Drawing for the job (mm, zero at the part's lowest x, y, z). Round coordinates to 2 decimals unless told otherwise and drop trailing zeros. Write each loop counter-clockwise with the first axis right and the second up, starting at its lowest first coordinate (ties: lowest second). Pieces come first, ordered by that corner, then holes. Notation, with made-up numbers: (38.5, 53) - (46.5, 53) arc R23 cw to (46.5, 69) - close; hole circle Ø9 at (35.25, -16.75). An arc over 180 degrees is marked (long way). Answer in a Markdown table with one row per item.
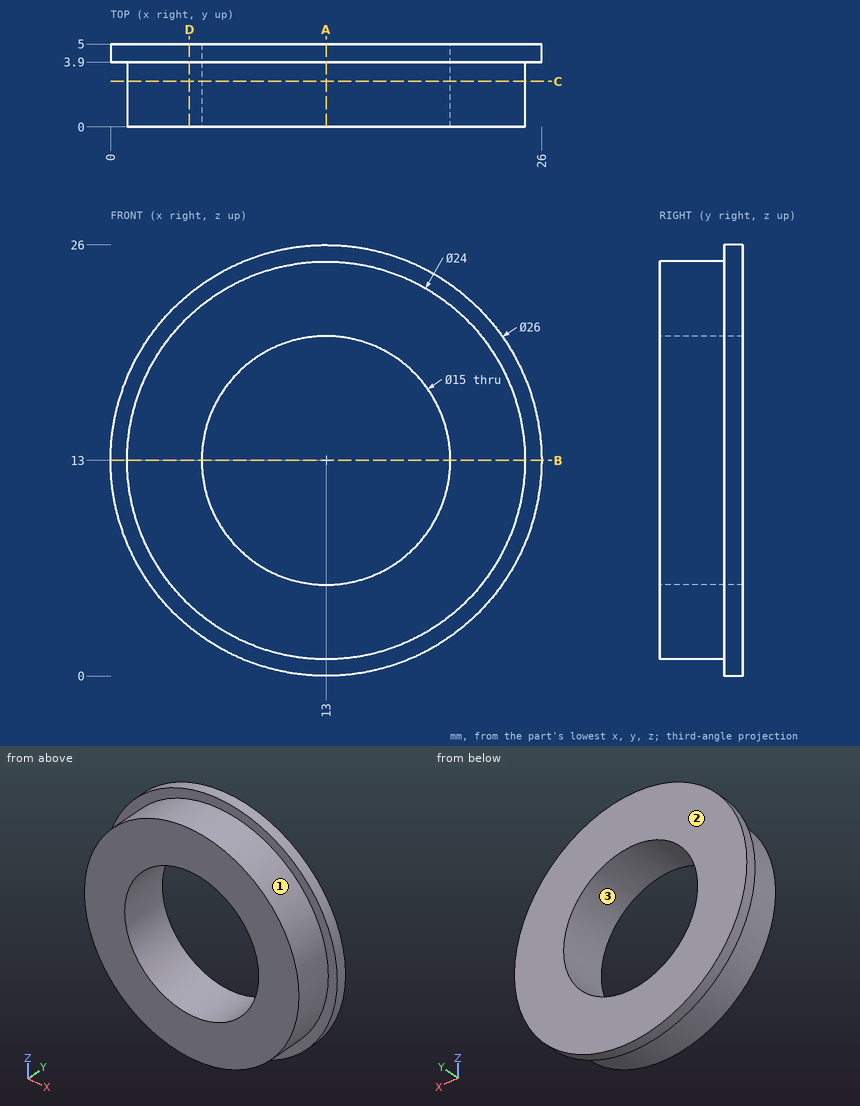
Q1. Flat gauge pins, fed straight in: pin 1 (3 mm diameter, centred on x = 17.5, y = 1.5, fed in from -Z); pin 2 (2 mm diameter, centred on y = 1, z = 21.5, fed in from +X); pin 3 (3 mm diameter, centred on y = 0.5, z = 15.5, fed in from +X). Where does each tip first touch, or does it go through?
Computed:
| item | result |
|---|---|
| pin 1 | stops at z = 1.38 |
| pin 2 | stops at x = 22.37 |
| pin 3 | stops at x = 24.96 |
Q2. Drill centre lines: line 1 (Z direction, x = 13, y = 1.2); line 2 (Z direction, x = 16, y = 4.75); line 3 (X direction, y = 4.8, z = 8.25). Where is each one in solid material? Low to high.
Computed:
| item | result |
|---|---|
| line 1 | z = 1 to 5.5, 20.5 to 25 |
| line 2 | z = 0.35 to 6.13, 19.87 to 25.65 |
| line 3 | x = 0.9 to 7.2, 18.8 to 25.1 |
Q3. Pull direction X, two halves, no side cores. Call the marked faces 1, 2 and 3: released by +X, released by -X, zero draft, split by the parting line, or undercut.
Computed:
| item | result |
|---|---|
| face 1 | split by the parting line |
| face 2 | zero draft |
| face 3 | undercut |
Q4. Saw through at C-C on y = 2.75. List the corners of the cut face in (x, z), then the cut area to 3 significant figures.
Computed:
| item | result |
|---|---|
| outline | circle Ø24 at (13, 13); hole circle Ø15 at (13, 13) |
| area | 276 mm2 |
Q5. Saw through at D-D on x = 4.75. List the corners of the cut face in (y, z).
Computed:
| item | result |
|---|---|
| outline | (0, 4.29) - (3.9, 4.29) - (3.9, 2.95) - (5, 2.95) - (5, 23.05) - (3.9, 23.05) - (3.9, 21.71) - (0, 21.71) - close |
Q6. Saw through at A-A on x = 13. List the corners of the cut face in (y, z), then the cut area to 3 significant figures.
Computed:
| item | result |
|---|---|
| outline | (0, 1) - (3.9, 1) - (3.9, 0) - (5, 0) - (5, 5.5) - (0, 5.5) - close; (0, 20.5) - (5, 20.5) - (5, 26) - (3.9, 26) - (3.9, 25) - (0, 25) - close |
| area | 47.2 mm2 |
Q7. Saw through at B-B on z = 13. List the corners of the cut face in (x, y).
Computed:
| item | result |
|---|---|
| outline | (0, 3.9) - (1, 3.9) - (1, 0) - (5.5, 0) - (5.5, 5) - (0, 5) - close; (20.5, 0) - (25, 0) - (25, 3.9) - (26, 3.9) - (26, 5) - (20.5, 5) - close |
